Here's how the part is built. I have some questions about the finished solid (model axes, mm). A direction names the side the tool comes from. Round coordinates to 2 decimals unless told otherwise and drop trailing zeros. Loops run counter-clockwise (first coordinate to the right, second up) from the corner with the lowest first, then second, coordinate; pieces in that order, holes last. Notation, with made-up numbers: M -9.75,78 L 30.25,78 A24 cw 30.25,92 Z; hole C 66,-24.5 d3. An arc over 180 degrees is marked long. Use a Markdown table: item, result.
Autodesk Inventor part; units mm, degrees
ref_plane "YZ Plane" through (0, 0, 0) normal (1, 0, 0) x (0, 1, 0)
ref_plane "XZ Plane" through (0, 0, 0) normal (0, 1, 0) x (-1, 0, 0)
ref_plane "XY Plane" through (0, 0, 0) normal (0, 0, 1) x (1, 0, 0)
sketch "Sketch1" plane through (0, 0, 0) normal (0, 0, 1) x (1, 0, 0)
  line L0 (0, -4.462) -> (0, 3.322)
  line L1 (3.05, 2.21) -> (3.05, 0.71)
  line L2 (3.05, 0.71) -> (1.5, 0.71)
  line L3 (1.5, 0.71) -> (1.5, -0.35)
  line L4 (1.5, -0.35) -> (2.925, -0.35)
  line L5 (2.925, -0.35) -> (2.925, -3.35)
  line L6 (2.925, -3.35) -> (4, -3.35)
  line L7 (4, -3.35) -> (4, 0)
  line L8 (4, 0) -> (6, 0)
  line L9 (6, 0) -> (6, 1.8)
  line L10 (6, 1.8) -> (3.5, 1.8)
  line L11 (3.5, 1.8) -> (3.5, 2.21)
  line L12 (3.5, 2.21) -> (3.05, 2.21)
  line L13 (-1.2, 0) -> (7.2, 0) construction
  point P0 (0, 0)
  dimension "d1" = 5.85
  dimension "d2" = 3
  dimension "d3" = 5.56
  dimension "d4" = 1.5
  dimension "d5" = 6.1
  dimension "d6" = 7
  dimension "d7" = 8
  dimension "d8" = 1.8
  dimension "d9" = 3.35
  dimension "d10" = 12
  dimension "d20" = 3
revolve "Revolution1" add sketch "Sketch1" angle 360 about axis through (0, -10, 0) along (0, 1, 0)
fillet "Fillet1" radius 1 1 edges at (-4, 0, 0)
sketch "Sketch2" plane through (0, 0, 0) normal (0, 0, 1) x (1, 0, 0)
  line L0 (-3.05, 2.21) -> (3.05, 2.21) construction
  line L1 (-3.5, 2.21) -> (3.5, 2.21) construction
  line L2 (-3.5, 1.8) -> (3.5, 1.8) construction
  line L3 (-6, 1.8) -> (6, 1.8) construction
  line L4 (3.4965, 2.21) -> (4.2066, 1.8)
  line L5 (4.2066, 1.8) -> (3.4965, 1.8)
  line L6 (3.4965, 1.8) -> (3.4965, 2.21)
  point P0 (0, 0)
  dimension "d13" = 0.0035
  dimension "d14" = 60
extrude "Extrusion1" add sketch "Sketch2" along normal mid plane 0.3
pattern_circular "Circular Pattern1" count 8 over 360 about axis through (0, -10, 0) along (0, 1, 0) of "Extrusion1"
sketch "Sketch3" plane through (0, 0, 0) normal (0, 1, 0) x (-1, 0, 0)
  line L0 (-4.3493, 7.0069) -> (-2.4607, 17.5268)
  arc A0 (2.4607, 17.5268) -> (-2.4607, 17.5268) centre (0, 17.085) ccw
  line L1 (2.4607, 17.5268) -> (4.3493, 7.0069)
  line L2 (8.4, 0) -> (-8.4, 0) construction
  line L3 (0, -10.4993) -> (0, 20.9956) construction
  line L4 (-4.25, 7.56) -> (4.25, 7.56) construction
  arc A1 (3.9598, 3.9598) -> (-3.9598, 3.9598) centre (0, 0) ccw
  arc A2 (4.3493, 7.0069) -> (4.7977, 4.7977) centre (6.2407, 6.2407) ccw
  arc A3 (-4.7977, 4.7977) -> (-4.3493, 7.0069) centre (-6.2407, 6.2407) ccw
  line L5 (0, 0) -> (6.2407, 6.2407) construction
  line L6 (3.6956, 5.8998) -> (6.4334, 3.1621) construction
  line L7 (-4.2, 7.1075) -> (-4.2, 5.2789) construction
  line L8 (4.2, 7.1509) -> (4.2, 5.2556) construction
  line L9 (4.7977, 4.7977) -> (3.9598, 3.9598)
  line L10 (-4.7977, 4.7977) -> (-3.9598, 3.9598)
  point P0 (0, 7.56)
  point P1 (0, 13.91)
  point P2 (0, 10.735)
  dimension "d21" = 17.085
  dimension "d22" = 5
  dimension "d23" = 9.525
  dimension "d25" = 8.5
  dimension "d26" = 5.6
  dimension "d29" = 3.175
  dimension "d30" = 3.175
  dimension "d38" = 45
  dimension "d40" = 6.785
  dimension "d41" = 8.4
extrude "Extrusion2" add sketch "Sketch3" along normal up to surface (1.8 mm away)
hole "Hole1" at (0, 0, 7.56) at (0, 0, 17.085) at (0, 0, 13.91) at (0, 0, 10.735) direction (0, 1, 0) diameter 1.6 end through all
pattern_circular "Circular Pattern2" count 4 over 360 about axis through (0, -10, 0) along (0, 1, 0) of "Extrusion2", "Hole1"
properties part number "4-PRONG SERVO ARM ONYX" material "Nylon 6/6"
Q1. For faces 4 (the cylindrical face through (-3.047, 1.45, 0.134)), 5 (the cylindrical face through (4.238, 0.887, 5.851)), which set-ups out of +Z, -Z, +X, -X, +Y, -Y let a thin tool reach every point of the face, with its end or its side?
Return value:
| item | result |
|---|---|
| face 4 | +Y |
| face 5 | +X, +Y, -Y |
Q2. I need wall thicknesses on line 1 (Z direction, x = 0, y = -2) (3 decimals); line 2 (X direction, y = 1, z = -7.56); line 3 (Y direction, x = -1.5, z = -5). Which ranges of each line are inside material? Lowest first, please. Write a range as from..to.
Return value:
| item | result |
|---|---|
| line 1 | z = -4..-2.925, 2.925..4 |
| line 2 | x = -4.25..-0.8, 0.8..4.25 |
| line 3 | y = 0..1.8 |
Q3. Imagine slicing it at B-B, the plane x = -7.56. Please give me the cut outline in (y, z).
Return value:
| item | result |
|---|---|
| outline | M 0,-4.25 L 1.8,-4.25 L 1.8,-0.8 L 0,-0.8 Z; M 0,0.8 L 1.8,0.8 L 1.8,4.25 L 0,4.25 Z |
Q4. Will these pins go through, and if not, where does the flat tip stop? P1, Ø2.5, axis at x = 0, z = 7.56, coming from the +Y side; P2, Ø1, axis at x = -10.735, z = 0, coming from the -Y side; P3, Ø1, axis at x = -7.5, z = -4.5, coming from the -Y side.
Return value:
| item | result |
|---|---|
| P1 | stops at y = 1.8 |
| P2 | passes through |
| P3 | stops at y = 0 |
Q5. Imagine slicing it at C-C, the plane y = -2.85. Please give me the cut outline in (x, z) (3 decimals), then the cut area to 3 significant figures.
Return value:
| item | result |
|---|---|
| outline | C 0,0 d8; hole C 0,0 d5.85 |
| area | 23.4 mm^2 |
Q6. Imagine slicing it at A-A, the plane z = -7.56. Please give me the cut outline in (x, y), then the cut area to 3 significant figures.
Return value:
| item | result |
|---|---|
| outline | M -4.25,0 L -0.8,0 L -0.8,1.8 L -4.25,1.8 Z; M 0.8,0 L 4.25,0 L 4.25,1.8 L 0.8,1.8 Z |
| area | 12.4 mm^2 |
Q7. We'd pull the mould along X, two halves only. Please class faces 1 (the flat face through (12.19, 0.89, -3.42)), 2 (the flat face through (1.3, -0.35, 1.3)), 3 (the flat face through (-12.19, 0.89, 3.42)): pulls with the +X half, pulls with the -X half, needs draft (parallel to the pull), parting line crosses it, or undercut.
Return value:
| item | result |
|---|---|
| face 1 | pulls with the +X half |
| face 2 | undercut |
| face 3 | pulls with the -X half |
